```python
from build123d import *

# Parameters (mm, degrees)
SKETCH_1_R               = 49
EXTRUDE_1_DEPTH          = 30
SKETCH_16_R              = 250
SKETCH_16_5_R            = 250
SKETCH_14_OUTSIDE_W      = 643.93
SKETCH_14_OUTSIDE_H      = 643.93
CUT_EXTRUDE_1_DEPTH      = 355.823900134
CUT_EXTRUDE_1_DEPTH_BACK = 355.823900134
SHELL_1_T                = 4
SKETCH_15_OUTSIDE_W      = 604.606
SKETCH_15_OUTSIDE_H      = 202.606
CUT_EXTRUDE_2_DEPTH      = 257.517055963
CUT_EXTRUDE_2_DEPTH_BACK = 257.517055963


with BuildPart() as part:
    # 草图1 → 凸台-拉伸1 (new, symmetric)
    with BuildSketch(Plane(origin=(0, 0, 0), x_dir=(1, 0, 0), z_dir=(0, 1, 0))):
        with Locations(Location((0, 0, 0), (0, 0, 270))):
            Circle(SKETCH_1_R)
    extrude(amount=EXTRUDE_1_DEPTH, both=True)

    # 草图16 → section 0 of loft_1
    with BuildSketch(Plane(origin=(0, 0, 0), x_dir=(1, 0, 0), z_dir=(0, 1, 0)), mode=Mode.PRIVATE) as loft_1_s0:
        Circle(SKETCH_16_R)
    # loft up to a face of the part (loft_1)
    loft([loft_1_s0.sketch, Face(Wire([part.edges().sort_by_distance((35.719462744, 30, -33.542808191))[0]]))])

    # 草图16<5> → section 0 of loft_3
    with BuildSketch(Plane(origin=(0, 0, 0), x_dir=(1, 0, 0), z_dir=(0, 1, 0)), mode=Mode.PRIVATE) as loft_3_s0:
        Circle(SKETCH_16_5_R)
    # loft up to a face of the part (loft_3)
    loft([loft_3_s0.sketch, Face(Wire([part.edges().sort_by_distance((-35.719462744, -30, -33.542808191))[0]]))])

    # 草图14 outside → 切除-拉伸1 (cut, two sides)
    with BuildSketch(Plane(origin=(0, 0, 0), x_dir=(1, 0, 0), z_dir=(0, 1, 0))) as cut_extrude_1_sk:
        Rectangle(SKETCH_14_OUTSIDE_W, SKETCH_14_OUTSIDE_H)
        with BuildLine():
            Line((-250, 0), (-9.604, -48.049590883))
            ThreePointArc((-9.604, -48.049590883), (0, -49), (9.604, -48.049590883))
            Line((9.604, -48.049590883), (250, 0))
            Line((250, 0), (9.604, 48.049590883))
            ThreePointArc((9.604, 48.049590883), (1.6e-08, 49), (-9.603999968, 48.049590889))
            Line((-9.603999968, 48.049590889), (-250, 0))
        make_face(mode=Mode.SUBTRACT)
    extrude(amount=CUT_EXTRUDE_1_DEPTH, mode=Mode.SUBTRACT)
    extrude(cut_extrude_1_sk.sketch, amount=-CUT_EXTRUDE_1_DEPTH_BACK, mode=Mode.SUBTRACT)

    # 抽壳1 (no face opened: a closed hollow body)
    add(offset(amount=-SHELL_1_T, mode=Mode.PRIVATE), mode=Mode.SUBTRACT)

    # 草图15 outside → 切除-拉伸2 (cut, two sides)
    with BuildSketch(Plane(origin=(0, 0, 0), x_dir=(1, 0, 0), z_dir=(0, 1, 0))) as cut_extrude_2_sk:
        Rectangle(SKETCH_15_OUTSIDE_W, SKETCH_15_OUTSIDE_H)
        with BuildLine():
            Line((-9.60400022, -48.049590839), (-164.621347882, -17.065214498))
            Line((-164.621347882, -17.065214498), (-164.621347882, 17.065214498))
            Line((-164.621347882, 17.065214498), (-9.604, 48.049590883))
            ThreePointArc((-9.604, 48.049590883), (0, 49), (9.604, 48.049590883))
            Line((9.604, 48.049590883), (165, 16.989530712))
            Line((165, 16.989530712), (165, -16.989530712))
            Line((165, -16.989530712), (9.604, -48.049590883))
            ThreePointArc((9.604, -48.049590883), (-1.12e-07, -49), (-9.60400022, -48.049590839))
        make_face(mode=Mode.SUBTRACT)
    extrude(amount=CUT_EXTRUDE_2_DEPTH, mode=Mode.SUBTRACT)
    extrude(cut_extrude_2_sk.sketch, amount=-CUT_EXTRUDE_2_DEPTH_BACK, mode=Mode.SUBTRACT)


solid = part.part
```
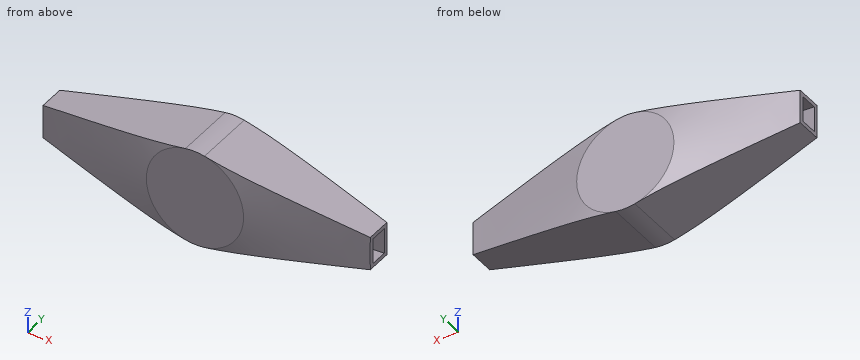
The model under review builds one solid part; all positions refer to its coordinate system, in mm. Coordinates: 2 decimals unless noted, no trailing zeros. Write each loop counter-clockwise with the first axis right and the second up, starting at its lowest first coordinate (ties: lowest second). Pieces come first, ordered by that corner, then holes.
1) We need section B-B on y = -22. State the section outline as (x, z) points.
2) Clearance check with flat-ended pins moving along their axes: pin 1 Ø4 at (x, y) = (-93.5, 23) entering from -Z; pin 2 Ø2 at (x, y) = (98.5, -9) entering from -Z; pin 3 Ø8 at (x, z) = (88.5, 31) entering from -Y. State where each tip first meets the part, or that it passes through.
3) To check wall thickness, follow probe 1 along Y at (x, z) = (39, 10); probe 2 along Z at (x, y) = (123, 2.5); probe 3 along Z at (x, y) = (-100, 21). State the ranges of each line that lie inside material, in increasing order.
4) We need section A-A on y = -4.5. State the section outline as (x, z) points, then the cut area to 3 significant figures.
Answer list:
1. outline: (-98, -30.38) - (-9.6, -48.05) arc R49 ccw to (9.6, -48.05) - (98, -30.38) arc R102.6 ccw to (98, 30.38) - (9.6, 48.05) arc R49 ccw to (-9.6, 48.05) - (-98, 30.38) arc R102.6 ccw to start; hole (-68.27, -32.24) - (-8.82, -44.13) arc R45 ccw to (8.82, -44.13) - (68.27, -32.24) arc R75.5 ccw to (68.27, 32.24) - (8.82, 44.13) arc R45 ccw to (-8.82, 44.13) - (-68.27, 32.24) arc R75.5 ccw to start
2. pin 1: stops at z = -31.68
2. pin 2: stops at z = -30.48
2. pin 3: stops at y = -23.91
3. probe 1: y = -30 to -26, 26 to 30
3. probe 2: z = -25.38 to -21.31, 21.31 to 25.38
3. probe 3: z = -29.98 to 29.98
4. outline: (-164.62, -17.07) - (-9.6, -48.05) arc R49 ccw to (9.6, -48.05) - (165, -16.99) - (165, -12.91) - (8.82, -44.13) arc R45 cw to (-8.82, -44.13) - (-164.62, -12.99) - close; (-164.62, 12.99) - (-8.82, 44.13) arc R45 cw to (8.82, 44.13) - (165, 12.91) - (165, 16.99) - (9.6, 48.05) arc R49 ccw to (-9.6, 48.05) - (-164.62, 17.07) - close
4. area: 2,690 mm2
